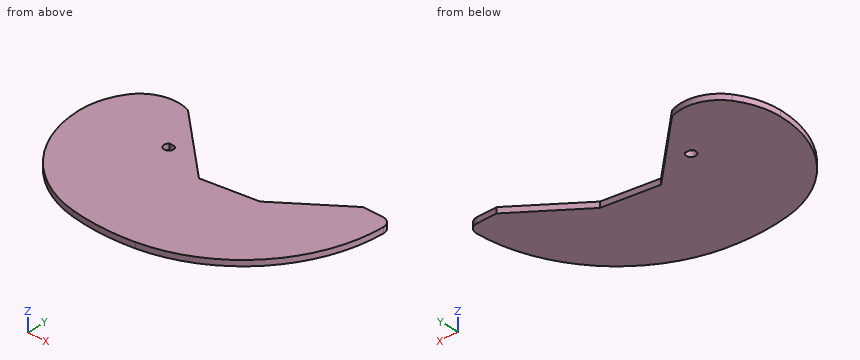
Autodesk Inventor part; units mm, degrees
ref_plane "YZ Plane" through (0, 0, 0) normal (1, 0, 0) x (0, 1, 0)
ref_plane "XZ Plane" through (0, 0, 0) normal (0, 1, 0) x (-1, 0, 0)
ref_plane "XY Plane" through (0, 0, 0) normal (0, 0, 1) x (1, 0, 0)
sketch "Sketch1" plane through (0, 0, 0) normal (0, 0, 1) x (1, 0, 0)
  line L0 (0, 0) -> (100, 0)
  arc A0 (100.0128, -3.6299) -> (100, 0) centre (-17.3055, -2.2293) ccw
  arc A1 (35.4459, -78.2987) -> (100.0128, -3.6299) centre (23.4974, -2.7164) ccw
  arc A2 (2.3748, -78.2085) -> (35.4459, -78.2987) centre (19.1908, 24.5253) ccw
  arc A3 (-43.4089, -24.3214) -> (2.3748, -78.2085) centre (11.1953, -24.3214) ccw
  arc A4 (-37.0013, -3.4804) -> (-43.4089, -24.3214) centre (-6.3121, -24.3214) ccw
  line L1 (84.6864, 0) -> (52.1966, -24.3214)
  line L2 (52.1966, -24.3214) -> (23.4974, -28.3171)
  line L3 (23.4974, -28.3171) -> (-12.0135, 4.2661)
  arc A5 (-12.0135, 4.2661) -> (-37.0013, -3.4804) centre (-19.6547, -15.2605) ccw
  point P0 (3.9425, 17.9592)
  dimension "d14" = 100
extrude "Extrusion1" add sketch "Sketch1" along normal blind 3
sketch "Sketch2" plane through (0, 0, 3) normal (0, 0, 1) x (1, 0, 0)
  arc A0 (-1.5, -18) -> (1.5, -18) centre (0, -20) ccw
  line L0 (-1.5, -18) -> (1.5, -18)
  point P0 (0, 0)
  dimension "d5" = 5
  dimension "d6" = 20
  dimension "d7" = 2
extrude "Extrusion2" cut sketch "Sketch2" against normal blind 3
fillet "Fillet7" radius 5 1 edges at (100, 0, 1.5)
properties part number "cam3"
Input: part model. Units: mm. Frame: model coordinates. Coordinates: 2 decimals unless noted, no trailing zeros. Order: outer loops, then holes, each group sorted by start corner. A loop starts at its lowest first (then second) coordinate and runs counter-clockwise, first axis right, second up. Notation, with made-up numbers: (-2, -0.75) - (9, -0.75) arc R20 cw to (9, 20.25) - close; hole circle Ø5 at (-26, -37). An arc over 180 degrees is marked (long way). Put each result on its own line as item: value.
1. Cut plane D-D on y = -42.5. Return the cut outline in (x, z).
Report:
outline: (-40.29, 0) - (88.86, 0) - (88.86, 3) - (-40.29, 3) - close
2. Cut plane A-A on x = 0. Return the cut outline in (y, z).
Report:
outline: (-77.77, 0) - (-22.5, 0) - (-22.5, 3) - (-77.77, 3) - close; (-18, 0) - (-6.76, 0) - (-6.76, 3) - (-18, 3) - close
3. Contact query for flat-ended pins moving along their axis: pin 1 Ø1 at (y, z) = (-21, 0.5) entering from -X; pin 2 Ø8 at (x, y) = (-28.5, -68.5) entering from +Z; pin 3 Ø6 at (x, y) = (0, -20) entering from +Z; pin 4 Ø1.5 at (x, z) = (-0.5, 1.5) entering from -Y. Output: stop coordinate, or through.
Report:
pin 1: stops at x = -43.3
pin 2: passes through
pin 3: stops at z = 3
pin 4: stops at y = -77.82
4. Line query: line 1 along X through (y, z) = (-20, 1.05); line 2 along X through (y, z) = (-15, 2); line 3 along X through (y, z) = (-5, 2.1). Output: solid intervals per line, ascending.
Report:
line 1: x = -43.16 to -2.5, 2.5 to 14.43, 57.97 to 98.04
line 2: x = -42.22 to 8.98, 64.65 to 99.03
line 3: x = -37.98 to -1.91, 78.01 to 99.98
5. Cut plane B-B on y = -20. Return the cut outline in (x, z), then the cut area to 3 significant figures.
Report:
outline: (-43.16, 0) - (-2.5, 0) - (-2.5, 3) - (-43.16, 3) - close; (2.5, 0) - (14.43, 0) - (14.43, 3) - (2.5, 3) - close; (57.97, 0) - (98.04, 0) - (98.04, 3) - (57.97, 3) - close
area: 278 mm2
6. Cut plane C-C on x = 86.5. Return the cut outline in (y, z).
Report:
outline: (-46.15, 0) - (0, 0) - (0, 3) - (-46.15, 3) - close
